Check sheet for the drawn part. Datum: minimum x, y, z corner. Units: mm. A direction names the side the tool comes from. Give positions to 0.01 mm unless a question says otherwise; leave off trailing zeros. Loops run counter-clockwise (first coordinate to the right, second up) from the corner with the lowest first, then second, coordinate; pieces in that order, holes last.
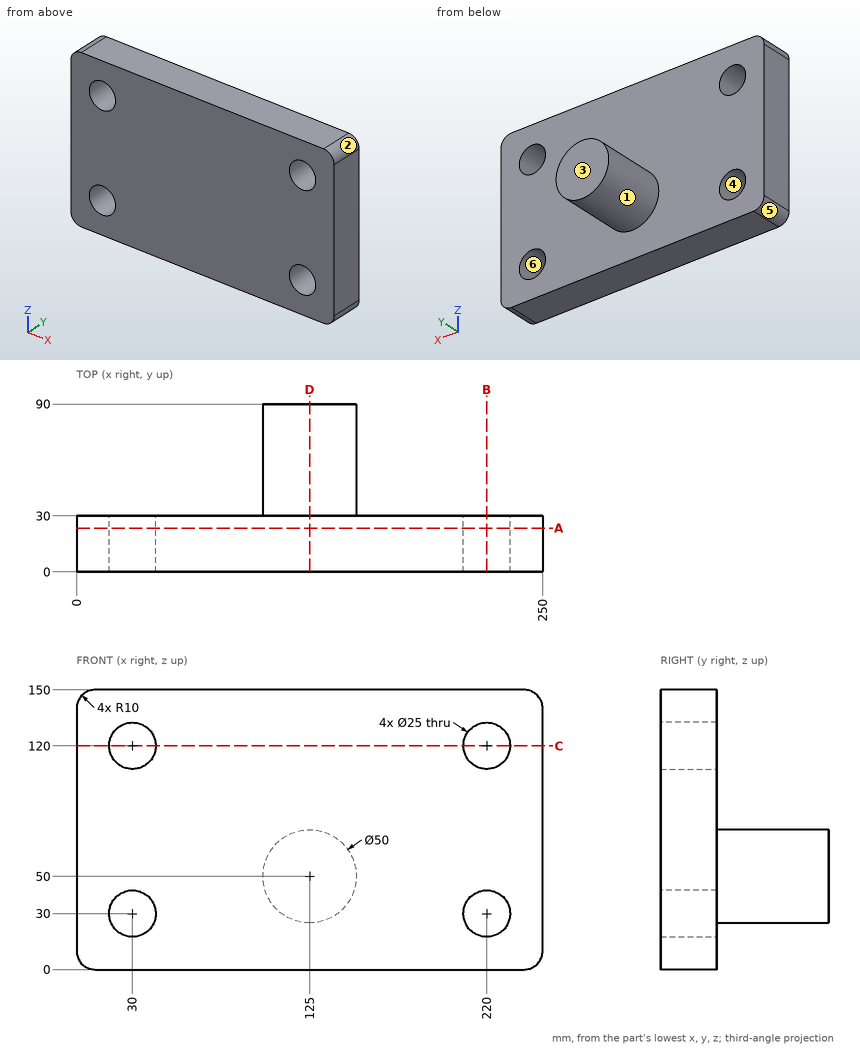
1) Sectioned sample at D-D on x = 125. Enter the section's corners in (y, z).
2) Sectioned sample at A-A on y = 23.5. Enter the section's corners in (x, z).
3) Mould release check, pull along Z, two halves, no side actions. Record for the marked faces 3, 4, 5 and 6: +Z half, -Z half, draft (parallel to the pull), parting line (faces both ways), or undercut.
4) Sectioned sample at B-B on x = 220. Enter the section's corners in (y, z), plus the area to 3 significant figures.
5) Tool access check on the marked faces 1 and 2. Record the directions out of +Z, -Z, +X, -X, +Y, -Y that give a thin tool (end or side, any length) a straight path to the whole face; none if there is none.
6) Sectioned sample at C-C on z = 120. Enter the section's corners in (x, y), plus the area to 3 significant figures.
7) Scan lines: line 1 along X through (y, z) = (23, 30); line 2 along X through (y, z) = (19, 24); line 3 along Y through (x, z) = (191, 113). Record each from-to range of solid material in increasing order.
8) Depth check by flat-ended pin: P1, Ø5, axis at y = 68, z = 42, coming from the -X side; P2, Ø8, axis at x = 151, z = 121.5, coming from the +Y side; P3, Ø20, axis at x = 30, z = 30, coming from the +Y side. Enter the tip coordinate at first touch or a pass-through.
Determined:
1. outline: (0, 0) - (30, 0) - (30, 25) - (90, 25) - (90, 75) - (30, 75) - (30, 150) - (0, 150) - close
2. outline: (0, 10) arc R10 ccw to (10, 0) - (240, 0) arc R10 ccw to (250, 10) - (250, 140) arc R10 ccw to (240, 150) - (10, 150) arc R10 ccw to (0, 140) - close; hole circle Ø25 at (30, 30); hole circle Ø25 at (30, 120); hole circle Ø25 at (220, 30); hole circle Ø25 at (220, 120)
3. face 3: draft
3. face 4: undercut
3. face 5: -Z half
3. face 6: undercut
4. outline: (0, 0) - (30, 0) - (30, 17.5) - (0, 17.5) - close; (0, 42.5) - (30, 42.5) - (30, 107.5) - (0, 107.5) - close; (0, 132.5) - (30, 132.5) - (30, 150) - (0, 150) - close
4. area: 3,000 mm2
5. face 1: +Y
5. face 2: +Z, +X, +Y, -Y
6. outline: (0, 0) - (17.5, 0) - (17.5, 30) - (0, 30) - close; (42.5, 0) - (207.5, 0) - (207.5, 30) - (42.5, 30) - close; (232.5, 0) - (250, 0) - (250, 30) - (232.5, 30) - close
6. area: 6,000 mm2
7. line 1: x = 0 to 17.5, 42.5 to 207.5, 232.5 to 250
7. line 2: x = 0 to 19.03, 40.97 to 209.03, 230.97 to 250
7. line 3: y = 0 to 30
8. P1: stops at x = 100.61
8. P2: stops at y = 30
8. P3: passes through
